Could you check a few things on this model? Use its own coordinates, in mm. A direction names the side the tool comes from. Give positions to 0.01 mm unless a question says otherwise; leave off trailing zeros. Write each loop counter-clockwise with the first axis right and the second up, starting at its lowest first coordinate (ties: lowest second). Pieces come first, ordered by that corner, then holes. Notation, with made-up numbers: (86.25, 42) - (117.25, 42) arc R18 cw to (117.25, 48) - close; hole circle Ø1 at (25.5, 61). An arc over 180 degrees is marked (long way). Use one line per item in the form item = value.
```python
from build123d import *

# Parameters (mm, degrees)
F0_W      = 70
F0_H      = 100
F1_DEPTH  = 50
F2_T      = -1.6
F3_W      = 10
F3_H      = 10
F4_DEPTH  = 70.001
F5_W      = 10
F5_H      = 10
F5_R      = 2
F6_DEPTH  = 1.6
F7_R      = 4.99999
F8_W      = 25
F8_H      = 15
F9_DEPTH  = 50.001
F10_W     = 25
F10_H     = 15
F11_DEPTH = 100.001


# Not quite as in the source:
# - a fillet or chamfer is up to 0.001 mm smaller than in the source, because OpenCascade refuses the exact size


with BuildPart() as f1:
    # F0 (on Top) → F1 (new body)
    with BuildSketch(Plane.XY):
        Rectangle(F0_W, F0_H)
    extrude(amount=F1_DEPTH)

    # F2
    f2_openings = [f1.faces().sort_by_distance(p)[0] for p in [
        (0, 0, 0),
    ]]
    offset(amount=F2_T, openings=f2_openings)

    # F3 (on face) → F4 (cut, through all)
    with BuildSketch(Plane.YZ.offset(35)):
        with Locations((45, 5)):
            Rectangle(F3_W, F3_H)
    extrude(amount=-F4_DEPTH, mode=Mode.SUBTRACT)

    # F5 (on Top) → F6 (join)
    with BuildSketch(Plane.XY):
        with Locations((40, 0)):
            Rectangle(F5_W, F5_H)
        with Locations((40, 0)):
            Circle(F5_R, mode=Mode.SUBTRACT)
        with Locations((-40, 0)):
            Rectangle(F5_W, F5_H)
        with Locations((-40, 0)):
            Circle(F5_R, mode=Mode.SUBTRACT)
        with Locations((-25, -55)):
            Rectangle(F5_W, F5_H)
        with Locations((-25, -55)):
            Circle(F5_R, mode=Mode.SUBTRACT)
        with Locations((25, -55)):
            Rectangle(F5_W, F5_H)
        with Locations((25, -55)):
            Circle(F5_R, mode=Mode.SUBTRACT)
    extrude(amount=F6_DEPTH)

    # F7 (radius 5 in the source; OpenCascade refuses exactly that, so slightly less here)
    f7_edges = [f1.edges().sort_by_distance(p)[0] for p in [
        (-45, -5, 0.8),
        (-45, 5, 0.8),
        (45, -5, 0.8),
        (45, 5, 0.8),
        (-30, -60, 0.8),
        (-20, -60, 0.8),
        (20, -60, 0.8),
        (30, -60, 0.8),
    ]]
    fillet(f7_edges, radius=F7_R)

    # F8 (on face) → F9 (cut, through all)
    with BuildSketch(Plane.XY.offset(50)):
        with Locations((0, 42.5)):
            Rectangle(F8_W, F8_H)
    extrude(amount=-F9_DEPTH, mode=Mode.SUBTRACT)

    # F10 (on face) → F11 (cut, through all)
    with BuildSketch(Plane.XZ.offset(50)):
        with Locations((0, 7.5)):
            Rectangle(F10_W, F10_H)
    extrude(amount=-F11_DEPTH, mode=Mode.SUBTRACT)


solid = f1.part
```
1. If we mould it in two halves opening along Y, with no side actions, what happens to faces 5 (the face through (-43, 4, 1)), 6 (the face through (-42, 0, 1)), 7 (the face through (-34, -17, 0))? For each: pulls with the +Y half, pulls with the -Y half, needs draft (parallel to the pull), parting line crosses it, or undercut.
Response values:
face_5 = pulls with the +Y half
face_6 = undercut
face_7 = needs draft
2. Imagine slicing it at D-D, the plane z = 24. List the corners of the cut face in (x, y) for me.
Response values:
outline = (-35, -50) - (35, -50) - (35, 50) - (12.5, 50) - (12.5, 48.4) - (33.4, 48.4) - (33.4, -48.4) - (-33.4, -48.4) - (-33.4, 48.4) - (-12.5, 48.4) - (-12.5, 50) - (-35, 50) - close
3. Imagine slicing it at B-B, the plane x = -14.5. List the corners of the cut face in (y, z) for me.
Response values:
outline = (-50, 0) - (-48.4, 0) - (-48.4, 48.4) - (48.4, 48.4) - (48.4, 10) - (50, 10) - (50, 50) - (-50, 50) - close
4. If I drill on line 1 (X direction, y = 16, z = 48); line 2 (Y direction, x = -19.5, z = 24.5); line 3 (Y direction, x = -12, z = 18), over which ranges is the centre line in solid material (lowest first)? Write a range as from..to.
Response values:
line_1 = -35..-33.4, 33.4..35
line_2 = -50..-48.4, 48.4..50
line_3 = -50..-48.4
5. Which directions (+Z, -Z, +X, -X, +Y, -Y) give clear straight access to the entire face, cutting with the end or side of a thin tool? Please do faces 1 (the face through (-21, -58, 1)), 2 (the face through (-33.4, -1, 24)), 3 (the face through (37.7, 0.1, 1.6)), 4 (the face through (-12.5, 49, 35)).
Response values:
face_1 = +Z, -Z, -Y
face_2 = -Z
face_3 = +Z, +X, +Y, -Y
face_4 = +Z, -Z, +Y
6. Imagine slicing it at A-A, the plane z = 5.5. List the corners of the cut face in (x, y) for me.
Response values:
outline = (-35, -50) - (-12.5, -50) - (-12.5, -48.4) - (-33.4, -48.4) - (-33.4, 40) - (-35, 40) - close; (12.5, -50) - (35, -50) - (35, 40) - (33.4, 40) - (33.4, -48.4) - (12.5, -48.4) - close
7. Imagine slicing it at C-C, the plane y = -7. List the corners of the cut face in (x, z) for me, and give its area (3 significant figures).
Response values:
outline = (-35, 0) - (-33.4, 0) - (-33.4, 48.4) - (33.4, 48.4) - (33.4, 0) - (35, 0) - (35, 50) - (-35, 50) - close
area = 267 mm²
8. For pin 1 (10 mm diameter, centred on x = -22.5, y = -35, fed in from -Z); pin 2 (1.8 mm diameter, centred on x = -38, z = 1, fed in from -Y); pin 3 (0.8 mm diameter, centred on y = -49, z = 7.5, fed in from +X), each with a flat end and sliding along its axis, tell me the tip position at first contact or that it passes through.
Response values:
pin_1 = 48.4
pin_2 = -5
pin_3 = 35
